For this review, take the finished solid that the model builds, in its own axes (mm). Face numbers are marked on the shaded views. A direction names the side the tool comes from. Coordinates: 2 decimals unless noted, no trailing zeros. Loops run counter-clockwise (first coordinate to the right, second up) from the corner with the lowest first, then second, coordinate; pieces in that order, holes last. Notation, with made-up numbers: M 5.5,73.5 L 38.5,73.5 A29 ccw 38.5,94.5 Z; hole C 24,70.5 d9. An arc over 180 degrees is marked long. Answer as a JSON object with one key per item and string values. Group by question number.
Item 1: Mouldability with a two-part tool opening along Z and no side actions: class the marked faces 3, 4, 5 and 6 as +Z half, -Z half, draft (parallel to the pull), parting line (faces both ways), or undercut.
Item 2: Wall thickness on L1, parallel to Y at x = 5, z = -3.75; L2, parallel to Y at x = 0.9, z = -42: over which ranges is each line inside the solid? List them lowest first. Write a range as from..to.
Item 3: Tool access review of the marked faces 1 and 2: name each direction out of +Z, -Z, +X, -X, +Y, -Y from which nothing blocks a thin tool from reaching the whole face with its end or side.
Item 4: Insertion check: pin 1 (3 mm diameter, centred on x = 9, z = -17, fed in from -Y); pin 2 (3.5 mm diameter, centred on x = 8, z = -58, fed in from -Y); pin 3 (4.5 mm diameter, centred on y = 15, z = -50.5, fed in from -X); pin 4 (3 mm diameter, centred on y = 15, z = -38.5, fed in from +X). Each pin has a flat end and moves straight along its axis. Give the tip position at first contact, or say it passes through.
Item 5: Add section C-C (y = 9). State the section outline as (x, z) points.
Item 6: Add section B-B (z = -63.5). State the section outline as (x, y) points.
Item 7: Add section A-A (z = -42). State the section outline as (x, y) points, then the cut area to 3 significant figures.
Item 8: Add section D-D (z = -28). State the section outline as (x, y) points, then the cut area to 3 significant figures.
Autodesk Inventor part; units mm, degrees
ref_plane "YZ Plane" through (0, 0, 0) normal (1, 0, 0) x (0, 1, 0)
ref_plane "XZ Plane" through (0, 0, 0) normal (0, 1, 0) x (-1, 0, 0)
ref_plane "XY Plane" through (0, 0, 0) normal (0, 0, 1) x (1, 0, 0)
sketch "Sketch1" plane through (0, 0, 0) normal (1, 0, 0) x (0, 1, 0)
  line L0 (0, 0) -> (28, 0)
  line L1 (28, 0) -> (28, -70)
  line L2 (28, -70) -> (0, -70)
  line L3 (0, -70) -> (0, 0)
  dimension "d20" = 70
extrude "Extrusion1" add sketch "Sketch1" along normal blind 13
sketch "Sketch2" plane through (13, 0, 0) normal (1, 0, 0) x (0, 0, -1)
  line L0 (0, 8) -> (0, 0)
  line L1 (0, 28) -> (0, 0)
  line L2 (0, 0) -> (70, 0)
  line L3 (0, 0) -> (70, 0)
  line L4 (70, 0) -> (70, 8)
  line L5 (70, 0) -> (70, 28)
  line L6 (0, 8) -> (70, 8)
extrude "Extrusion2" cut sketch "Sketch2" against normal blind 10
sketch "Sketch3" plane through (13, 0, 0) normal (1, 0, 0) x (0, 0, -1)
  line L0 (70, 0) -> (0, 0)
  line L1 (70, 0) -> (42, 0)
  line L2 (42, 0) -> (42, 15)
  circle A0 centre (42, 15) radius 12.5
  dimension "d21" = 28
  dimension "d22" = 15
  dimension "d23" = 25
extrude "Extrusion3" cut sketch "Sketch3" against normal blind 10
sketch "Sketch4" plane through (3, 0, 0) normal (1, 0, 0) x (0, 0, -1)
  arc A0 (52.3562, 8) -> (31.6438, 8) centre (42, 15) ccw
  circle A1 centre (42, 15) radius 3.5
  line L0 (42, 15) -> (50.5, 15)
  line L1 (42, 15) -> (33.5, 15)
  circle A2 centre (33.5, 15) radius 1.7
  circle A3 centre (50.5, 15) radius 1.7
  point P0 (0, 0)
  dimension "d24" = 7
  dimension "d25" = 8.5
  dimension "d26" = 8.5
  dimension "d68" = 3.4
  dimension "d69" = 3.4
extrude "Extrusion4" cut sketch "Sketch4" against normal blind 3
sketch "Sketch5" plane through (0, 0, -70) normal (0, 0, -1) x (-1, 0, 0)
  line L0 (0, 28) -> (-13, 28)
  line L1 (0, 28) -> (-5, 28)
  line L2 (-5, 28) -> (-5, 23)
  line L3 (-5, 23) -> (0, 23)
  line L4 (0, 23) -> (0, 28)
  line L5 (0, 8) -> (-5, 8)
  line L6 (-5, 8) -> (-5, 13)
  line L7 (-5, 13) -> (0, 13)
  line L8 (0, 13) -> (0, 8)
  point P0 (0, 0)
  dimension "d29" = 5
  dimension "d30" = 5
  dimension "d31" = 5
  dimension "d32" = 5
hole "Hole1" at (5, 13, -70) at (5, 23, -70) direction (0, 0, 1) diameter 2.4638 depth 10 tip angle 118
sketch "Sketch6" plane through (0, 0, 0) normal (0, 0, 1) x (1, 0, 0)
  line L0 (0, 28) -> (13, 28)
  circle A0 centre (5, 23) radius 1.2319
  line L1 (0, 28) -> (5, 28)
  line L2 (5, 28) -> (5, 23)
  line L3 (5, 23) -> (0, 23)
  line L4 (0, 23) -> (0, 28)
  circle A1 centre (5, 13) radius 1.2319
  line L5 (0, 8) -> (5, 8)
  line L6 (5, 8) -> (5, 13)
  line L7 (5, 13) -> (0, 13)
  line L8 (0, 13) -> (0, 8)
  point P0 (0, 0)
  point P1 (3.8741, 22.5)
  point P2 (6.1259, 22.5)
hole "Hole2" at (5, 23, 0) at (5, 13, 0) direction (0, 0, -1) diameter 2.4638 depth 10 tip angle 118
sketch "Sketch9" plane through (3, 8, 0) normal (0, -1, 0) x (1, 0, 0)
  line L0 (-3, 0) -> (10, 0)
  line L1 (10, 0) -> (5, 0)
  line L2 (5, 0) -> (5, -15)
  line L3 (5, -15) -> (10, -15)
  line L4 (10, -15) -> (10, 0)
  line L5 (10, -70) -> (10, 0)
  line L6 (10, -70) -> (5, -70)
  line L7 (5, -70) -> (5, -58)
  line L8 (5, -58) -> (10, -58)
  line L9 (10, -58) -> (10, -70)
  dimension "d70" = 5
  dimension "d71" = 15
  dimension "d74" = 5
  dimension "d75" = 12
hole "Hole4" at (8, 8, -15) at (8, 8, -58) direction (0, 1, 0) diameter 4.1402 depth 10 tip angle 118
properties part number "mocowanie silnika"
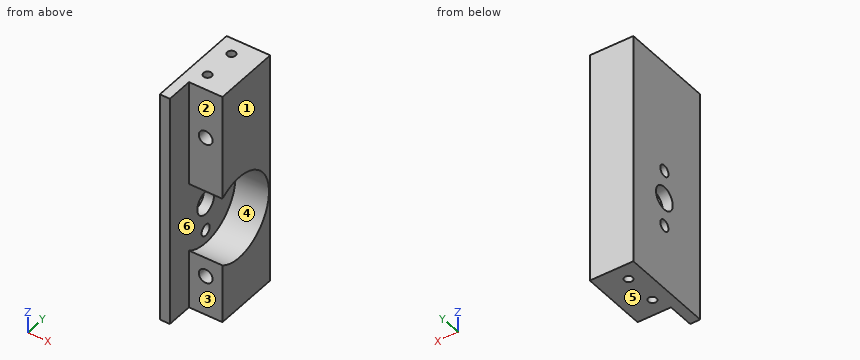
From the geometry:
{
 "1": {"face 3": "draft", "face 4": "undercut", "face 5": "-Z half", "face 6": "undercut"},
 "2": {"L1": "y = 8..11.77, 14.23..21.77, 24.23..28", "L2": "y = 0..11.5, 18.5..28"},
 "3": {"face 1": "+Z, -Z, +X, +Y, -Y", "face 2": "+Z, -Z, +X, -Y"},
 "4": {"pin 1": "stops at y = 8", "pin 2": "stops at y = 18.19", "pin 3": "stops at x = 0", "pin 4": "stops at x = 3"},
 "5": {"outline": "M 0,-70 L 13,-70 L 13,-52.97 L 3,-52.97 L 3,-31.03 L 13,-31.03 L 13,0 L 0,0 Z; hole C 8,-58 d4.14; hole C 8,-15 d4.14"},
 "6": {"outline": "M 0,0 L 3,0 L 3,8 L 13,8 L 13,28 L 0,28 Z; hole C 5,13 d2.46; hole C 5,23 d2.46"},
 "7": {"outline": "M 0,0 L 3,0 L 3,11.5 L 0,11.5 Z; M 0,18.5 L 3,18.5 L 3,27.5 L 13,27.5 L 13,28 L 0,28 Z", "area": "68.0 mm²"},
 "8": {"outline": "M 0,0 L 3,0 L 3,8 L 13,8 L 13,28 L 0,28 Z", "area": "284 mm²"}
}
